Autodesk Inventor part; units mm, degrees
ref_plane "YZ Plane" through (0, 0, 0) normal (1, 0, 0) x (0, 1, 0)
ref_plane "XZ Plane" through (0, 0, 0) normal (0, 1, 0) x (-1, 0, 0)
ref_plane "XY Plane" through (0, 0, 0) normal (0, 0, 1) x (1, 0, 0)
sketch "Sketch1" plane through (0, 0, 0) normal (0, 1, 0) x (-1, 0, 0)
  circle A0 centre (0, 0) radius 3.5
  circle A1 centre (0, 0) radius 10
  line L0 (0, 0) -> (-7.5, 0) construction
  line L1 (0, 0) -> (0, 3.5) construction
  line L2 (0, 3.5) -> (0, 10) construction
  point P0 (-5, 0)
  point P1 (-7.5, 3.5)
  point P2 (-5, 2.5)
  point P3 (0, 4.75)
  dimension "d0" = 7
  dimension "d2" = 20
  dimension "d3" = 7.5
  dimension "d47" = 5
  dimension "d50" = 3.5
  dimension "d57" = 2.5
  dimension "d62" = 4.75
extrude "Extrusion1" add sketch "Sketch1" along normal blind 1.6 contours A0 | A1
extrude "Extrusion2" add sketch "Sketch1" against normal blind 2.7 and the other way blind 2 contours A0
hole "Hole2" at (0, -2.7, 0) direction (0, 1, 0) diameter 3 end through all
hole "Hole3" at (0, -2.7, 0) direction (0, 1, 0) diameter 5 depth 2.2
hole "Hole5" at (0, 2, 0) direction (0, -1, 0) diameter 5 depth 0.8
hole "Hole6" at (7.5, 0, 0) at (5, 0, 0) at (7.5, 0, 3.5) at (5, 0, 2.5) direction (0, 1, 0) diameter 1.5 end through all
mirror "Mirror1" about plane through (0, 0, 0) normal (1, 0, 0) of "Hole6"
hole "Hole7" at (0, 0, 4.75) direction (0, 1, 0) diameter 1 end through all
pattern_linear "Rectangular Pattern1" count 3 spacing 1.75 along (0, 0, 1) of "Hole7"
mirror "Mirror2" about plane through (0, 0, 0) normal (0, 0, 1) of "Hole6", "Mirror1", "Hole7", "Rectangular Pattern1"
properties part number "servo arm DS939HV round"
Verification items for the finished model (mm, model axes). A direction names the side the tool comes from. Give positions to 0.01 mm unless a question says otherwise; leave off trailing zeros. Order: outer loops, then holes, each group sorted by start corner. A loop starts at its lowest first (then second) coordinate and runs counter-clockwise, first axis right, second up. Notation, with made-up numbers: M 6.25,6 L 59.25,6 A18 ccw 59.25,31 Z; hole C -19,-4.75 d8. An arc over 180 degrees is marked long. Answer as a JSON object with one key per item and string values. Group by question number.
1) Cross-section at D-D (z = 0). Give the number of separate pieces and of enclosed holes in the cut face, then the cut area to 3 significant figures.
2) Cross-section at A-A (z = -6.5). Enter the section's corners in (x, y), then the cut area to 3 significant figures.
3) Cross-section at C-C (y = -1.9). Enter the section's corners in (x, z).
4) Mould release check, pull along X, two halves, no side actions. Record for faces 4 (the face through (5.732, 0.811, 0.163)), 5 (the face through (2.17, 0.79, 9.76)), 6 (the face through (-4, 0, -2)): released by +X, released by -X, zero draft, split by the parting line, or undercut.
5) Access from +Z, -Z, +X, -X, +Y, -Y to the whole of each face (thin tool, end or side, straight path). Record for faces 1 (the face through (0, -0.5, -2)), 2 (the face through (2.44, 1.59, -0.54)), 3 (the face through (-2, -2.7, -2)).
6) Scan lines: line 1 along Z through (x, y) = (7.5, 0.05); line 2 along X through (y, z) = (0.3, 3.5); line 3 along Y through (x, z) = (6, 6.75). Record each from-to range of solid material in increasing order. Write a range as [from, to].
7) Cross-section at B-B (x = 7.5). Enter the section's corners in (y, z).
8) Depth check by flat-ended pin: pin 1 Ø3 at (x, z) = (-5, 6) entering from +Y; pin 2 Ø3 at (x, z) = (5, -7) entering from -Y; pin 3 Ø1.2 at (x, z) = (7.5, -3.5) entering from +Y; pin 4 Ø4 at (x, z) = (0, 0) entering from -Y. Enter the tip coordinate at first touch or a pass-through.
Result sheet:
{
 "1": {"separate pieces": "6", "enclosed holes": "0", "area": "24.0 mm2"},
 "2": {"outline": "M -7.6,0 L -0.5,0 L -0.5,1.6 L -7.6,1.6 Z; M 0.5,0 L 7.6,0 L 7.6,1.6 L 0.5,1.6 Z", "area": "22.7 mm2"},
 "3": {"outline": "C 0,0 d7; hole C 0,0 d5"},
 "4": {"face 4": "undercut", "face 5": "split by the parting line", "face 6": "zero draft"},
 "5": {"face 1": "-Y", "face 2": "+Y", "face 3": "+Z, -Z, +X, -X, -Y"},
 "6": {"line 1": "z = [-6.61, -4.25], [-2.75, -0.75], [0.75, 2.75], [4.25, 6.61]", "line 2": "x = [-9.37, -8.25], [-6.75, 6.75], [8.25, 9.37]", "line 3": "y = [0, 1.6]"},
 "7": {"outline": "M 0,-6.61 L 1.6,-6.61 L 1.6,-4.25 L 0,-4.25 Z; M 0,-2.75 L 1.6,-2.75 L 1.6,-0.75 L 0,-0.75 Z; M 0,0.75 L 1.6,0.75 L 1.6,2.75 L 0,2.75 Z; M 0,4.25 L 1.6,4.25 L 1.6,6.61 L 0,6.61 Z"},
 "8": {"pin 1": "stops at y = 1.6", "pin 2": "stops at y = 0", "pin 3": "passes through", "pin 4": "stops at y = -0.5"}
}
